```python
from build123d import *

# Parameters (mm, degrees)
F0_W     = 7.578362
F0_H     = 80.447212
F1_DEPTH = 5.08
F2_W     = 52.174097
F2_H     = 3.789182
F2_W_2   = 41.680984
F2_H_2   = 3.789179
F3_DEPTH = 5.08
F4_DEPTH = 5.08
F6_DEPTH = 5.08


with BuildPart() as f1:
    # F0 (on Front) → F1 (new body)
    with BuildSketch(Plane.XZ):
        with Locations((-0.291475, 3.934916)):
            Rectangle(F0_W, F0_H)
    extrude(amount=F1_DEPTH)

    # F2 (on Front) → F3 (join)
    with BuildSketch(Plane.XZ):
        with Locations((-0.437214, 37.017377)):
            Rectangle(F2_W, F2_H)
        with Locations((-0.437213, 29.730491)):
            Rectangle(F2_W_2, F2_H_2)
    extrude(amount=F3_DEPTH)

    # F2 (on Front) → F4 (join)
    with BuildSketch(Plane.XZ):
        with Locations((-0.437214, 37.017377)):
            Rectangle(F2_W, F2_H)
        with Locations((-0.437213, 29.730491)):
            Rectangle(F2_W_2, F2_H_2)
    extrude(amount=F4_DEPTH)

    # F5 (on Front) → F6 (join)
    with BuildSketch(Plane.XZ):
        Polygon((20.986229, 19.09164), (-20.111803, 5.683771), (-20.111803, 2.477542), (20.986229, 15.885411), align=None)
    extrude(amount=F6_DEPTH)


solid = f1.part
```
Model file for the job. Use its own axes, mm. A direction names the side the tool comes from. Coordinates: 2 decimals unless noted, no trailing zeros. Order: outer loops, then holes, each group sorted by start corner. A loop starts at its lowest first (then second) coordinate and runs counter-clockwise, first axis right, second up. Notation, with made-up numbers: (-29, 60.5) -> (-6, 60.5) arc R7 cw to (-6, 70.5) -> close; hole circle Ø2 at (69.25, 37.25). An arc over 180 degrees is marked (long way). Answer as a JSON object with one key per item and string values. Group by question number.
1) Cut at D-D, the plane z = -16. Write the cut outline in (x, y).
2) Flat gauge pins, fed straight in: pin 1 (1.5 mm diameter, centred on y = -1.5, z = 41.5, fed in from +X); pin 2 (5 mm diameter, centred on x = -4, z = 7, fed in from +Y); pin 3 (3 mm diameter, centred on y = -2, z = 33.5, fed in from -X); pin 4 (1 mm diameter, centred on y = -3, z = 5, fed in from -X). Where does each tip first touch, or does it go through?
3) Cut at B-B, the plane y = -2.45. Write the cut outline in (x, z).
4) Cut at A-A, the plane z = 14.5. Write the cut outline in (x, y).
5) Pull direction Z, two halves, no side cores. Call faces 5 (the face through (14, -3, 35.123)), 6 (the face through (14, -3, 38.912)), 7 (the face through (-4.081, -3, 41)), 8 (the face through (-12.208, -2.504, 5.056)): +Z half, -Z half, draft (parallel to the pull), parting line (faces both ways), or undercut.
6) Drill centre lines: L1, parallel to Z at x = 5.5, y = -4.8; L2, parallel to Z at x = -6.5, y = -3.95; L3, parallel to X at y = -4.65, z = 25.5. Where is each one in solid material? Low to high.
7) Cut at C-C, the plane x = 7. Write the cut outline in (y, z).
8) Which spindle directions (+Z, -Z, +X, -X, +Y, -Y) get a long thin tool onto all of the face, cutting with end or side? Do faces 1 (the face through (3.498, -3, -13)), 2 (the face through (-4.081, -3, 19)), 3 (the face through (12.364, -2.504, 16.279)), 4 (the face through (3.498, -3, 33)). Say none if no direction does.
Check values:
{
 "1": {"outline": "(-4.08, -5.08) -> (3.5, -5.08) -> (3.5, 0) -> (-4.08, 0) -> close"},
 "2": {"pin 1": "stops at x = 3.5", "pin 2": "stops at y = 0", "pin 3": "stops at x = -4.08", "pin 4": "stops at x = -20.11"},
 "3": {"outline": "(-26.52, 35.12) -> (-4.08, 35.12) -> (-4.08, 31.63) -> (-21.28, 31.63) -> (-21.28, 27.84) -> (-4.08, 27.84) -> (-4.08, 10.91) -> (-20.11, 5.68) -> (-20.11, 2.48) -> (-4.08, 7.71) -> (-4.08, -36.29) -> (3.5, -36.29) -> (3.5, 10.18) -> (20.99, 15.89) -> (20.99, 19.09) -> (3.5, 13.39) -> (3.5, 27.84) -> (20.4, 27.84) -> (20.4, 31.63) -> (3.5, 31.63) -> (3.5, 35.12) -> (25.65, 35.12) -> (25.65, 38.91) -> (3.5, 38.91) -> (3.5, 44.16) -> (-4.08, 44.16) -> (-4.08, 38.91) -> (-26.52, 38.91) -> close"},
 "4": {"outline": "(-4.08, -5.08) -> (3.5, -5.08) -> (3.5, 0) -> (-4.08, 0) -> close; (6.91, -5.08) -> (16.74, -5.08) -> (16.74, 0) -> (6.91, 0) -> close"},
 "5": {"face 5": "undercut", "face 6": "+Z half", "face 7": "draft", "face 8": "-Z half"},
 "6": {"L1": "z = 10.83 to 14.04, 27.84 to 31.63, 35.12 to 38.91", "L2": "z = 6.92 to 10.12, 27.84 to 31.63, 35.12 to 38.91", "L3": "x = -4.08 to 3.5"},
 "7": {"outline": "(-5.08, 11.32) -> (0, 11.32) -> (0, 14.53) -> (-5.08, 14.53) -> close; (-5.08, 27.84) -> (0, 27.84) -> (0, 31.63) -> (-5.08, 31.63) -> close; (-5.08, 35.12) -> (0, 35.12) -> (0, 38.91) -> (-5.08, 38.91) -> close"},
 "8": {"face 1": "-Z, +X, +Y, -Y", "face 2": "-X, +Y, -Y", "face 3": "+Y, -Y", "face 4": "+X, +Y, -Y"}
}
